CAD build for the part. Positions are in the model's coordinates, mm. A direction names the side the tool comes from. Round coordinates to 2 decimals unless told otherwise and drop trailing zeros.
Autodesk Inventor part; units mm, degrees
ref_plane "YZ Plane" through (0, 0, 0) normal (1, 0, 0) x (0, 1, 0)
ref_plane "XZ Plane" through (0, 0, 0) normal (0, 1, 0) x (-1, 0, 0)
ref_plane "XY Plane" through (0, 0, 0) normal (0, 0, 1) x (1, 0, 0)
sketch "Skizze1" plane through (0, 0, 0) normal (0, 0, 1) x (1, 0, 0)
  arc A0 (-44.0908, 75) -> (44.0908, 75) centre (0, 0) ccw
  line L0 (-44.0908, 75) -> (44.0908, 75)
  dimension "d0" = 174
  dimension "d1" = 75
extrude "Extrusion1" add sketch "Skizze1" along normal blind 2
sketch "Skizze2" plane through (0, 0, 2) normal (0, 0, 1) x (1, 0, 0)
  arc A0 (-44.0908, 75) -> (44.0908, 75) centre (0, 0) ccw
  line L0 (44.0908, 75) -> (-44.0908, 75)
  arc A1 (-41.2795, 65) -> (41.2795, 65) centre (0, 0) ccw
  line L1 (-41.2795, 65) -> (41.2795, 65)
  dimension "d4" = 10
extrude "Extrusion2" add sketch "Skizze2" along normal blind 1
sketch "Skizze8" plane through (0, 0, 2) normal (0, 0, 1) x (1, 0, 0)
  line L0 (41.2795, 65) -> (-41.2795, 65)
  arc A0 (-41.2795, 65) -> (41.2795, 65) centre (0, 0) ccw
  circle A1 centre (0, 0) radius 80 construction
  circle A2 centre (-80, 0) radius 6.5
  circle A3 centre (80, 0) radius 6.5
  line L1 (-121.8, 0) -> (121.8, 0)
  dimension "d38" = 160
  dimension "d39" = 13
  dimension "d40" = 13
extrude "Extrusion4" add sketch "Skizze8" along normal blind 1 contours A3 L1 A0 | A0 L1 A3 | A2 L1 A0 | A0 L1 A2 | L1 A3 A0 | A0 A3 L1 | L1 A2 A0 | A0 A2 L1
sketch "Skizze3" plane through (0, 0, 3) normal (0, 0, 1) x (1, 0, 0)
  line L0 (0, 107.4) -> (0, -119.4)
  line L1 (-121.8, 0) -> (121.8, 0)
  point P0 (0, 0)
  point P1 (-80, 0)
  point P2 (80, 0)
  dimension "d7" = 160
hole "Bohrung1" at (-80, 0, 3) at (80, 0, 3) direction (0, 0, -1) diameter 4.4 end through all
sketch "Skizze4" plane through (0, 0, 3) normal (0, 0, 1) x (1, 0, 0)
  circle A0 centre (0, 0) radius 83 construction
  line L0 (0, 0) -> (-47.6068, 67.9896) construction
  line L1 (0, 0) -> (-63.5817, -53.3514) construction
  line L2 (0, 117) -> (0, -121)
  line L3 (-121.8, 0) -> (121.8, 0)
  point P0 (63.5817, -53.3514)
  point P1 (47.6068, 67.9896)
  dimension "d15" = 166
  dimension "d16" = 55
  dimension "d17" = 40
hole "Bohrung2" at (-63.5817, -53.3514, 3) at (-47.6068, 67.9896, 3) at (63.5817, -53.3514, 3) at (47.6068, 67.9896, 3) direction (0, 0, -1) diameter 2.75 end through all
sketch "Skizze5" plane through (0, 0, 0) normal (0, 0, -1) x (-1, 0, 0)
  line L0 (0, -119.4) -> (0, 107.4)
  line L1 (-121.8, 0) -> (121.8, 0)
  point P0 (0, 0)
  point P1 (-45, 28)
  point P2 (-27.5, -45.25)
  point P3 (45, 28)
  point P4 (27.5, -45.25)
  point P5 (0, 11.5)
  dimension "d113" = 45
  dimension "d114" = 28
  dimension "d115" = 27.5
  dimension "d116" = 45.25
  dimension "d117" = 11.5
hole "Bohrung3" at (45, 28, 0) at (27.5, -45.25, 0) at (0, 11.5, 0) at (-45, 28, 0) at (-27.5, -45.25, 0) direction (0, 0, 1) diameter 14 end through all
fillet "Rundung1" radius 2 4 edges at (-44.0908, 75, 1.5) (44.0908, 75, 1.5) (41.2795, 65, 2.5) (-41.2795, 65, 2.5)
sketch "Skizze17" plane through (0, 0, 0) normal (0, 0, -1) x (-1, 0, 0)
  line L0 (-43.5431, 75) -> (43.5431, 75)
  line L1 (28.5, 75) -> (-28.5, 75)
  line L2 (-28.5, 75) -> (-28.5, -28.5)
  line L3 (-28.5, -28.5) -> (28.5, -28.5)
  line L4 (28.5, -28.5) -> (28.5, 75)
  line L5 (0, -119.4) -> (0, 107.4)
  line L6 (-43.5431, 75) -> (43.5431, 75)
  line L7 (-30.5, 75) -> (30.5, 75)
  line L8 (30.5, 75) -> (30.5, -30.5)
  line L9 (30.5, -30.5) -> (-30.5, -30.5)
  line L10 (-30.5, -30.5) -> (-30.5, 75)
  point P0 (0, 0)
  point P1 (-5, 75)
  dimension "d107" = 28.5
  dimension "d108" = 57
  dimension "d109" = 2
  dimension "d110" = 2
extrude "Extrusion10" cut sketch "Skizze17" against normal blind 1 contours L0 L2 L3 L5 L9 L10 | L5 L3 L4 L0 L8 L9
chamfer "Fase1" distance 0.3 angle 45 17 edges at (-27.5, -52.25, 0) (27.5, -52.25, 0) (-45, 21, 0) (45, 21, 0) (0, 4.5, 0) (-63.5817, -51.9764, 0) (63.5817, -51.9764, 0) (-47.6068, 69.3646, 0) (47.6068, 69.3646, 0) (-80, 2.2, 0) (80, 2.2, 0) (0, -87, 0) (44.0745, 74.9281, 0) (37.0215, 75, 0) (-44.0745, 74.9281, 0) (-37.0215, 75, 0) (0, 75, 0)
chamfer "Fase2" distance 0.5 angle 45 7 edges at (-27.5, -52.25, 2) (27.5, -52.25, 2) (-45, 21, 2) (0, 4.5, 2) (45, 21, 2) (-80, 2.2, 3) (80, 2.2, 3)
sketch "Skizze15" plane through (0, 0, 0) normal (0, 0, -1) x (-1, 0, 0)
  circle A0 centre (0, 0) radius 25
  circle A1 centre (54.772, 35) radius 20
  circle A2 centre (35, -54.772) radius 20
  circle A3 centre (-35, -54.772) radius 20
  circle A4 centre (-54.772, 35) radius 20
  line L0 (0, -119.4) -> (0, 107.4)
  line L1 (-121.8, 0) -> (121.8, 0)
  circle A5 centre (-54.772, 35) radius 20.5
  circle A6 centre (-35, -54.772) radius 20.5
  circle A7 centre (54.772, 35) radius 20.5
  circle A8 centre (35, -54.772) radius 20.5
  circle A9 centre (0, 0) radius 25.5
  dimension "d91" = 50
  dimension "d92" = 40
  dimension "d93" = 40
  dimension "d94" = 40
  dimension "d95" = 40
  dimension "d96" = 35
  dimension "d97" = 54.772
  dimension "d98" = 54.772
  dimension "d99" = 35
  dimension "d100" = 41
  dimension "d101" = 41
  dimension "d102" = 41
  dimension "d103" = 41
  dimension "d104" = 51
extrude "Extrusion9" cut sketch "Skizze15" against normal blind 0.2 contours A5 | A6 | A7 | A8
equation "\"d110\" = d109"
equation "\"d98\" = d97"
equation "\"d99\" = d96"
properties part number "Gehäuse Unterplatte"
1. Drill centre lines: line 1 (Y direction, x = 0, z = 1.25); line 2 (X direction, y = -45.25, z = 0.6); line 3 (X direction, y = -17.5, z = 0.8). Where is each one in solid material? Low to high.
2. Pin check, flat tips, straight feed: P1, Ø1, axis at x = -16.5, z = 2.5, coming from the -Y side; P2, Ø8, axis at x = -22, y = 57, coming from the +Z side; P3, Ø1.5, axis at x = 43.5, z = 2, coming from the -Y side. Stop position of each tip, or through.
3. Cut at A-A, the plane y = 25. Give the number of separate pieces and of enclosed holes in the cut face, and give its area (3 significant figures).
4. Tool access for faces 1 (the face through (1.614, -76.983, 2.493)), 2 (the face through (-7, 66, 3)): list every direction of +Z, -Z, +X, -X, +Y, -Y with a clear straight run to the whole face (end or side of a thin tool).
5. Mould opens along Y. For faces 3 (the face through (-81.855, -1.183, 1.385)), 4 (the face through (-55, 35, 0)), 5 (the face through (-44, -73, 0.2)) say: released by +Y, released by -Y, zero draft, split by the parting line, or undercut.
Outcome:
1. line 1: y = -87 to 4.5, 18.5 to 75
1. line 2: x = -74.31 to -34.5, -20.5 to 20.5, 34.5 to 74.31
1. line 3: x = -85.22 to -30.5, -28.5 to 28.5, 30.5 to 85.22
2. P1: stops at y = -85.52
2. P2: stops at z = 2
2. P3: stops at y = -75.77
3. separate pieces: 3
3. enclosed holes: 0
3. area: 298 mm2
4. face 1: +Z
4. face 2: +Z, +X, -X, +Y, -Y
5. face 3: undercut
5. face 4: zero draft
5. face 5: undercut
